from build123d import *

# Parameters (mm, degrees)
F0_W          = 30
F0_H          = 56
F1_DEPTH      = 15
F1_DEPTH_BACK = 1
F2_START      = 7
F0_R          = 10
F2_DEPTH      = 8
F3_R          = 3
F4_R          = 3
F6_DEPTH      = 8
F7_T1_DEPTH   = 27.8062484749
F7_T3_DEPTH   = 27.8062484749
F9_DEPTH      = 30
F10_SIZE      = 2


# Not quite as in the source:
# - a fillet or chamfer that OpenCascade refuses, or shapes differently, is made with other operations: its cross-section is extruded or revolved along the edge and cut away or added


with BuildPart() as f1:
    # F0 (on Top) → F1 (new body, two sides)
    with BuildSketch(Plane.XY) as f1_sk:
        with Locations((0, 17.5)):
            Rectangle(F0_W, F0_H)
    extrude(amount=F1_DEPTH)
    extrude(f1_sk.sketch, amount=-F1_DEPTH_BACK)

    # F0 (on Top) → F2 (join)
    with BuildSketch(Plane.XY.offset(F2_START)):
        with BuildLine():
            Line((15, -40.5), (15, -10.5))
            Line((15, -10.5), (-15, -10.5))
            Line((-15, -10.5), (-15, -40.5))
            ThreePointArc((-15, -40.5), (-13.5355339059, -44.0355339059), (-10, -45.5))
            Line((-10, -45.5), (10, -45.5))
            ThreePointArc((10, -45.5), (13.5355339059, -44.0355339059), (15, -40.5))
        make_face()
        with Locations((0, -30.7424795181)):
            Circle(F0_R, mode=Mode.SUBTRACT)
    extrude(amount=F2_DEPTH)

    # F3
    f3_edges = [f1.edges().sort_by_distance(p)[0] for p in [
        (0, -10.5, 7),
        (0, -10.5, -1),
    ]]
    fillet(f3_edges, radius=F3_R)

    # F4
    f4_edges = [f1.edges().sort_by_distance(p)[0] for p in [
        (-10, -30.74248, 15),
        (-10, -30.74248, 7),
    ]]
    fillet(f4_edges, radius=F4_R)

    # F5 (on face) → F6 (cut)
    with BuildSketch(Plane.XZ.offset(45.5)):
        Polygon((10, 7), (0, 15), (-5, 15), (5, 7), align=None)
    extrude(amount=-F6_DEPTH, mode=Mode.SUBTRACT)

    # F7: fillet of radius 3 on 2 edges, made by hand

    # F7_s2 → F7_t1 (cut)
    with BuildSketch(Plane(origin=(-16.2223697294, 0, 12.9778957835), x_dir=(0, 1, 0), z_dir=(0.7808688094, 0, -0.6246950476))):
        with BuildLine():
            ThreePointArc((-45.5, 5.5895569039), (-44.6213203436, 7.7108772474), (-42.5, 8.5895569039))
            Line((-42.5, 8.5895569039), (-45.5, 8.5895569039))
            Line((-45.5, 8.5895569039), (-45.5, 5.5895569039))
        make_face()
    extrude(amount=F7_T1_DEPTH, mode=Mode.SUBTRACT)

    # F7_s4 → F7_t3 (cut)
    with BuildSketch(Plane(origin=(8.5394429001, 0, -6.8315543201), x_dir=(0, 1, 0), z_dir=(-0.7808688094, 0, 0.6246950476))):
        with BuildLine():
            ThreePointArc((-45.5, -14.7130321416), (-44.6213203436, -12.5917117981), (-42.5, -11.7130321416))
            Line((-42.5, -11.7130321416), (-45.5, -11.7130321416))
            Line((-45.5, -11.7130321416), (-45.5, -14.7130321416))
        make_face()
    extrude(amount=F7_T3_DEPTH, mode=Mode.SUBTRACT)

    # F8 (on face) → F9 (cut, through all)
    with BuildSketch(Plane(origin=(-15, 0, 0), x_dir=(0, -1, 0), z_dir=(-1, 0, 0))):
        Polygon((0, 5), (0, 11), (-40, 11), (-40, 10), (-40, 5), (-37, 5), (-37, -1), (-3, -1), (-3, 5), align=None)
    extrude(amount=-F9_DEPTH, mode=Mode.SUBTRACT)

    # F10
    f10_edges = [f1.edges().sort_by_distance(p)[0] for p in [
        (0, 37, 5),
        (0, 3, 5),
    ]]
    chamfer(f10_edges, length=F10_SIZE)


solid = f1.part
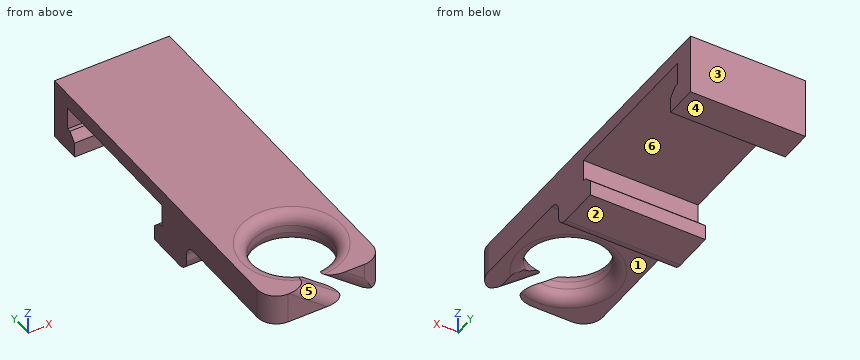
Input: part model. Units: mm. Frame: model coordinates. Face numbers are marked on the shaded views. A direction names the side the tool comes from. Coordinates: 2 decimals unless noted, no trailing zeros. Loops run counter-clockwise (first coordinate to the right, second up) from the corner with the lowest first, then second, coordinate; pieces in that order, holes last.
(1) First-contact query: pin 1 Ø6.5 at (x, z) = (4.5, 8.5) entering from -Y; pin 2 Ø12 at (x, y) = (0, -30.74) entering from +Z; pin 3 Ø6 at (x, y) = (5.5, 25.5) entering from -Z; pin 4 Ø4.5 at (x, z) = (-4, 1) entering from -Y. Flat tips, straight axial feed; report the tip coordinate or a pass-through.
(2) Pull-direction query (Y, two-part tool) for the marked faces 3, 4, 5 and 6; classes: released by +Y, released by -Y, zero draft, split by the parting line, or undercut.
(3) Material intervals for probe 1 along Y at (x, z) = (-7, 10.5); probe 2 along Y at (x, z) = (-7.5, 9.75); probe 3 along Y at (x, z) = (0, 11.45), sorted ascending.
(4) Set-up query: the marked faces 1 and 2. Return all of +Z, -Z, +X, -X, +Y, -Y with unobstructed straight access to the full face (end or side cutting, diameter ignored); none if empty.
(5) Section B-B on y = 27. Return the cut outline in (x, z), then the cut area to 3 significant figures.
(6) Section A-A on x = 2.5. Count the separate pieces of the cut face and the enclosed holes in it, then the cut area to 3 significant figures.
(7) Section C-C on y = -12.5. Return the cut outline in (x, z).
Data:
1. pin 1: stops at y = -45.37
1. pin 2: passes through
1. pin 3: stops at z = 11
1. pin 4: stops at y = -10.5
2. face 3: released by +Y
2. face 4: zero draft
2. face 5: released by -Y
2. face 6: undercut
3. probe 1: y = -45.5 to -37.88, -23.6 to 0, 40 to 45.5
3. probe 2: y = -45.5 to -37.37, -24.11 to 0, 40 to 45.5
3. probe 3: y = -20.74 to 45.5
4. face 1: -Z, +X, -X, -Y
4. face 2: -Z, +X, -X, +Y, -Y
5. outline: (-15, 11) - (15, 11) - (15, 15) - (-15, 15) - close
5. area: 120 mm2
6. separate pieces: 3
6. enclosed holes: 0
6. area: 540 mm2
7. outline: (-15, 6.83) - (15, 6.83) - (15, 15) - (-15, 15) - close
